from build123d import *

# Parameters (mm, degrees)
BOSS_EXTRU_1_DEPTH = 8
CONG_1_R           = 5
CONG_2_R           = 1


with BuildPart() as part:
    # Esquisse1 → Boss.-Extru.1 (new body)
    with BuildSketch(Plane.XY):
        with BuildLine():
            Line((0, 0), (0, 81))
            Line((0, 81), (12.878679656, 81))
            ThreePointArc((12.878679656, 81), (15, 81), (15, 83.121320344))
            Line((15, 83.121320344), (15, 89))
            Line((15, 89), (35, 89))
            Line((35, 89), (35, 83.121320344))
            ThreePointArc((35, 83.121320344), (35, 81), (37.121320344, 81))
            Line((37.121320344, 81), (50, 81))
            Line((50, 81), (0, 0))
        make_face()
    extrude(amount=BOSS_EXTRU_1_DEPTH)

    # Congé1
    cong_1_edges = [part.edges().sort_by_distance(p)[0] for p in [
        (0, 0, 4),
    ]]
    fillet(cong_1_edges, radius=CONG_1_R)

    # Congé2
    cong_2_edges = [part.edges().sort_by_distance(p)[0] for p in [
        (50, 81, 4),
    ]]
    fillet(cong_2_edges, radius=CONG_2_R)


solid = part.part
The listing builds one solid part. Answer for the finished solid, in the listing's coordinates (mm). A direction names the side the tool comes from. Round coordinates to 2 decimals unless told otherwise and drop trailing zeros. Loops run counter-clockwise (first coordinate to the right, second up) from the corner with the lowest first, then second, coordinate; pieces in that order, holes last. Notation, with made-up numbers: M -18,-16.75 L 36,-16.75 A30 ccw 36,8.25 Z; hole C 51.5,43 d9. An arc over 180 degrees is marked long. Return JSON: item names as keys, results as strings.
Q1. Find the intervals of material crossed by line 1 along Y through (x, z) = (5, 4.75); line 2 along X through (y, z) = (74, 1); line 3 along X through (y, z) = (83, 7), in increasing order. Write a range as from..to.
Results list:
{"line 1": "y = 12.62..81", "line 2": "x = 0..45.68", "line 3": "x = 15.11..34.89"}
Q2. Find section C-C, the plane y = 58. Determine the outline of the cut face in (x, z).
Results list:
{"outline": "M 0,0 L 35.8,0 L 35.8,8 L 0,8 Z"}
Q3. Find section A-A, the plane z = 2. Determine the outline of the cut face in (x, y).
Results list:
{"outline": "M 0,17.62 A5 ccw 9.25,14.99 L 49.06,79.47 A1 ccw 48.21,81 L 37.12,81 A1.5 cw 35,83.12 L 35,89 L 15,89 L 15,83.12 A1.5 cw 12.88,81 L 0,81 Z"}
Q4. Which of the six approach directions +Z, -Z, +X, -X, +Y, -Y give full straight-line access (tool end or side, diameter ignored) to faces 1 (the face through (15, 86, 4)), 2 (the face through (49.09, 80.47, 4.06)), 3 (the face through (43, 81, 4))?
Results list:
{"face 1": "+Z, -Z, -X, +Y", "face 2": "+Z, -Z, +X", "face 3": "+Z, -Z, +X, +Y"}
Q5. Find section B-B, the plane x = 38.5. Determine the outline of the cut face in (y, z), plus the area to 3 significant figures.
Results list:
{"outline": "M 62.37,0 L 81,0 L 81,8 L 62.37,8 Z", "area": "149 mm2"}
Q6. Each of these flat-tipped pins is pushed along its axis until it touches: pin 1 Ø12 at (x, y) = (31, 35) entering from -Z; pin 2 Ø4.5 at (y, z) = (85, 3.5) entering from +X; pin 3 Ø4 at (x, z) = (5, 5) entering from +Y; pin 4 Ø3 at (y, z) = (41, 5.5) entering from +X. Where does it stop, or does it pass through?
Results list:
{"pin 1": "passes through", "pin 2": "stops at x = 35", "pin 3": "stops at y = 81", "pin 4": "stops at x = 26.23"}
